Work out the finished part from the listing and answer in its coordinate system (mm). A direction names the side the tool comes from. Round coordinates to 2 decimals unless told otherwise and drop trailing zeros. Order: outer loops, then holes, each group sorted by start corner. A loop starts at its lowest first (then second) coordinate and runs counter-clockwise, first axis right, second up. Notation, with made-up numbers: (13, -11.5) - (46, -11.5) arc R31 ccw to (46, 13.5) - close; hole circle Ø11 at (64.5, 32). An arc over 180 degrees is marked (long way). Put each result on its own line as item: value.
```python
from build123d import *

# Parameters (mm, degrees)
SKETCH1_W             = 15
SKETCH1_H             = 13
SKETCH1_R             = 1.5
BOSS_EXTRUDE1_DEPTH   = 5
BOSS_EXTRUDE1_2_DEPTH = 5
SKETCH2_W             = 15
SKETCH2_H             = 3
BOSS_EXTRUDE2_DEPTH   = 43.35
SKETCH3_W             = 15
SKETCH3_H             = 19
BOSS_EXTRUDE3_DEPTH   = 3
BOSS_EXTRUDE5_START   = -15
SKETCH5_W             = 15
SKETCH5_H             = 19
BOSS_EXTRUDE5_DEPTH   = 3


with BuildPart() as part:
    # Sketch1 → Boss-Extrude1 (new body)
    with BuildSketch(Plane(origin=(0, 0, 0), x_dir=(0, 0, -1), z_dir=(1, 0, 0))):
        with Locations((7.5, 6.5)):
            Rectangle(SKETCH1_W, SKETCH1_H)
        with Locations((4.5, 5)):
            Circle(SKETCH1_R, mode=Mode.SUBTRACT)
        with Locations((10.5, 5)):
            Circle(SKETCH1_R, mode=Mode.SUBTRACT)
    extrude(amount=BOSS_EXTRUDE1_DEPTH)



with BuildPart() as body_2:
    # Sketch1 → Boss-Extrude1 2 (new body)
    with BuildSketch(Plane(origin=(0, 0, 0), x_dir=(0, 0, -1), z_dir=(1, 0, 0))):
        with Locations((7.5, 32.5)):
            Rectangle(SKETCH1_W, SKETCH1_H)
        with Locations((4.5, 34)):
            Circle(SKETCH1_R, mode=Mode.SUBTRACT)
        with Locations((10.5, 34)):
            Circle(SKETCH1_R, mode=Mode.SUBTRACT)
    extrude(amount=BOSS_EXTRUDE1_2_DEPTH)


with BuildPart() as part_1:
    add(part.part)

    add(body_2.part)  # Boss-Extrude2 merges body 2
    # Sketch2 → Boss-Extrude2 (add)
    with BuildSketch(Plane(origin=(5, 0, 0), x_dir=(0, 0, -1), z_dir=(1, 0, 0))):
        with Locations((7.5, 27.5)):
            Rectangle(SKETCH2_W, SKETCH2_H)
        with Locations((7.5, 11.5)):
            Rectangle(SKETCH2_W, SKETCH2_H)
    extrude(amount=BOSS_EXTRUDE2_DEPTH)

    # Sketch3 → Boss-Extrude3 (add)
    with BuildSketch(Plane(origin=(48.35, 0, 0), x_dir=(0, 0, -1), z_dir=(1, 0, 0))):
        with Locations((7.5, 19.5)):
            Rectangle(SKETCH3_W, SKETCH3_H)
    extrude(amount=BOSS_EXTRUDE3_DEPTH)

    # Sketch5 → Boss-Extrude5 (add)
    with BuildSketch(Plane(origin=(51.35, 0, 0), x_dir=(0, 0, -1), z_dir=(1, 0, 0)).offset(BOSS_EXTRUDE5_START)):
        with Locations((7.5, 19.5)):
            Rectangle(SKETCH5_W, SKETCH5_H)
    extrude(amount=-BOSS_EXTRUDE5_DEPTH)


solid = part_1.part
```
1) Given pin 1 Ø4.5 at (x, z) = (20.5, -9) entering from +Y; pin 2 Ø5 at (y, z) = (36, -4) entering from +X; pin 3 Ø4 at (x, z) = (28, -10) entering from -Y, each flat-ended and moving along its own axis, determine where each tip first touches the part or whether it passes through.
Findings below:
pin 1: stops at y = 29
pin 2: stops at x = 5
pin 3: stops at y = 10
2) For faces 4 (the flat face through (16, 13, -7)), 5 (the flat face through (42, 26, -7)), 6 (the flat face through (5, 34, -7)), determine the directions among +Z, -Z, +X, -X, +Y, -Y from which every point of the face is accessible in a straight line to the end or side of a thin tool.
Findings below:
face 4: +Z, -Z, -X
face 5: +Z, -Z
face 6: +Z, -Z, +X, +Y
3) A cutting plane is placed at A-A on z = -4.5. Write down the section's boundary in (x, y), then the cut area to 3 significant figures.
Findings below:
outline: (0, 0) - (5, 0) - (5, 3.5) - (0, 3.5) - close; (0, 6.5) - (5, 6.5) - (5, 10) - (51.35, 10) - (51.35, 29) - (5, 29) - (5, 32.5) - (0, 32.5) - (0, 26) - (33.35, 26) - (33.35, 13) - (0, 13) - close; (0, 35.5) - (5, 35.5) - (5, 39) - (0, 39) - close; hole (36.35, 13) - (48.35, 13) - (48.35, 26) - (36.35, 26) - close
area: 456 mm2
4) A cutting plane is placed at B-B on y = 5. Write down the section's boundary in (x, z), then the cut area to 3 significant figures.
Findings below:
outline: (0, -15) - (5, -15) - (5, -12) - (0, -12) - close; (0, -9) - (5, -9) - (5, -6) - (0, -6) - close; (0, -3) - (5, -3) - (5, 0) - (0, 0) - close
area: 45.0 mm2
5) A cutting plane is placed at D-D on y = 20.5. Write down the section's boundary in (x, z), then the cut area to 3 significant figures.
Findings below:
outline: (33.35, -15) - (36.35, -15) - (36.35, 0) - (33.35, 0) - close; (48.35, -15) - (51.35, -15) - (51.35, 0) - (48.35, 0) - close
area: 90.0 mm2
6) For a pull along X with two mould halves and no side action, classify faces 1 (the flat face through (22, 12, 0)), 2 (the flat face through (0, 7, -7)), 3 (the flat face through (42, 13, -7)) as pulls with the +X half, pulls with the -X half, needs draft (parallel to the pull), parting line crosses it, or undercut.
Findings below:
face 1: needs draft
face 2: pulls with the -X half
face 3: undercut
7) Straight lines are drawn through the part: L1, parallel to Y at x = 1.8, z = -4.5; L2, parallel to X at y = 23, z = -2.5; L3, parallel to Y at x = 33, z = -6. For each, find the intervals that lie inside material, in ascending order. Write a range as from..to.
Findings below:
L1: y = 0..3.5, 6.5..13, 26..32.5, 35.5..39
L2: x = 33.35..36.35, 48.35..51.35
L3: y = 10..13, 26..29
8) A cutting plane is placed at C-C on x = 40. Write down the section's boundary in (y, z).
Findings below:
outline: (10, -15) - (13, -15) - (13, 0) - (10, 0) - close; (26, -15) - (29, -15) - (29, 0) - (26, 0) - close
